Could you check a few things on this model? Use its own coordinates, in mm. Face numbers are marked on the shaded views. Round coordinates to 2 decimals unless told otherwise and drop trailing zeros. Write each loop counter-clockwise with the first axis right and the second up, starting at its lowest first coordinate (ties: lowest second). Pieces come first, ordered by that corner, then holes. Notation, with made-up numbers: (8, -19) -> (45, -19) arc R26 cw to (45, 15) -> close; hole circle Ø8 at (66, -34.75). An arc over 180 degrees is marked (long way). One line per question, with ' | ' between items. Start each with the question number.
1. Imagine slicing it at C-C, the plane x = 0. State how many separate pieces and enclosed holes the cut face has, and give its area (3 significant figures).
2. Imagine slicing it at D-D, the plane x = -7.75. List the corners of the cut face in (y, z) for me.
3. For pin 1 Ø4 at (x, y) = (-5, 25) entering from -Z; pin 2 Ø4 at (x, z) = (1.5, 22.5) entering from +Y; pin 3 Ø10 at (y, z) = (3.5, -17) entering from +X; pin 4 Ø2.5 at (x, z) = (0, 20) entering from +Y, each with a flat end and sliding along its axis, tell me the tip position at first contact or that it passes through.
4. Imagine slicing it at A-A, the plane z = 0. List the corners of the cut face in (x, y) for me (3 decimals), and give its area (4 significant figures).
5. Imagine slicing it at B-B, the plane y = 15.5. List the corners of the cut face in (x, z) for me.
6. If I drill on line 1 along Z through (x, y) = (0, 28.95) (3 decimals); line 2 along Z through (x, y) = (0, 2.2); line 3 along X through (y, z) = (4.5, -19), over which ranges is the centre line in solid material (lowest first)? Write a range as [from, to].
7. Thinking about a two-plate mould opening in Z: for the marked faces 1, 2, 3 and 4, which applies, released by +Z, released by -Z, zero draft, split by the parting line, or undercut?
Autodesk Inventor part; units mm, degrees
ref_plane "YZ Plane" through (0, 0, 0) normal (1, 0, 0) x (0, 1, 0)
ref_plane "XZ Plane" through (0, 0, 0) normal (0, 1, 0) x (-1, 0, 0)
ref_plane "XY Plane" through (0, 0, 0) normal (0, 0, 1) x (1, 0, 0)
sketch "スケッチ1" plane through (0, 0, 0) normal (0, 1, 0) x (-1, 0, 0)
  line L0 (0, 0) -> (0, -20) construction
  line L1 (0, 0) -> (0, 20) construction
  circle A0 centre (0, 20) radius 1.7
  circle A1 centre (0, -20) radius 1.7
  circle A2 centre (0, 20) radius 4.7
  circle A3 centre (0, -20) radius 4.7
  line L2 (4.698231, 19.871077) -> (4.7, -19.999792)
  line L3 (-4.697377, 19.843003) -> (-4.697377, -20.156997)
  circle A4 centre (0, 0) radius 12.5
  point P0 (-4.697377, 11.58381)
  point P1 (4.698599, 11.583314)
  point P2 (4.699627, -11.582897)
  point P3 (-4.697377, -11.58381)
  dimension "d0" = 20
  dimension "d1" = 20
  dimension "d2" = 3.4
  dimension "d3" = 3.4
  dimension "d5" = 3
  dimension "d6" = 3
  dimension "d7" = 25
sketch "スケッチ1 outline for 押し出し1" plane through (0, 0, 0) normal (0, 1, 0) x (-1, 0, 0)
  arc A0 (-4.697377, 11.58381) -> (4.698599, 11.583314) centre (0, 0) cw
  line L0 (-4.697377, 19.843003) -> (-4.697377, 11.58381)
  line L1 (4.698599, 11.583314) -> (4.698231, 19.871077)
  arc A1 (4.698231, 19.871077) -> (-4.697377, 19.843003) centre (0, 20) ccw
  circle A2 centre (0, 20) radius 1.7
  arc A3 (-4.697377, -20.156997) -> (4.7, -19.999792) centre (0, -20) ccw
  line L2 (-4.697377, -11.58381) -> (-4.697377, -20.156997)
  line L3 (4.7, -19.999792) -> (4.699627, -11.582897)
  arc A4 (4.699627, -11.582897) -> (-4.697377, -11.58381) centre (0, 0) cw
  circle A5 centre (0, -20) radius 1.7
extrude "押し出し1" add sketch "スケッチ1 outline for 押し出し1" along normal blind 5
sketch "スケッチ2" plane through (0, 5, 0) normal (0, 1, 0) x (1, 0, 0)
  line L0 (-4.698599, -11.583314) -> (-4.698231, -19.871077)
  arc A0 (-4.698231, -19.871077) -> (4.697377, -19.843003) centre (0, -20) ccw
  line L1 (4.697377, -19.843003) -> (4.697377, -11.58381)
  arc A1 (-4.698599, -11.583314) -> (4.697377, -11.58381) centre (0, 0) ccw
  circle A2 centre (0, -20) radius 1.7
  arc A3 (4.697377, 20.156997) -> (-4.7, 19.999792) centre (0, 20) ccw
  line L2 (-4.7, 19.999792) -> (-4.699627, 11.582897)
  arc A4 (4.697377, 11.58381) -> (-4.699627, 11.582897) centre (0, 0) ccw
  line L3 (4.697377, 11.58381) -> (4.697377, 20.156997)
  circle A5 centre (0, 20) radius 1.7
  circle A6 centre (0, 0) radius 16
  point P0 (4.697377, 15.294922)
  point P1 (-4.699791, 15.294181)
  point P2 (-4.698434, -15.294598)
  point P3 (4.697377, -15.294922)
  dimension "d10" = 32
extrude "押し出し2" add sketch "スケッチ2" along normal blind 20 contours A1 L1 A6 L0 | A6 L3 A4 L2
sketch "スケッチ3" plane through (0, 25, 0) normal (0, 1, 0) x (1, 0, 0)
  line L0 (-4.698599, -11.583314) -> (-4.698434, -15.294598)
  arc A0 (-4.698434, -15.294598) -> (4.697377, -15.294922) centre (0, 0) ccw
  line L1 (4.697377, -15.294922) -> (4.697377, -11.58381)
  arc A1 (-4.698599, -11.583314) -> (4.697377, -11.58381) centre (0, 0) ccw
  line L2 (-4.699791, 15.294181) -> (-4.699627, 11.582897)
  arc A2 (4.697377, 11.58381) -> (-4.699627, 11.582897) centre (0, 0) ccw
  line L3 (4.697377, 11.58381) -> (4.697377, 15.294922)
  arc A3 (4.697377, 15.294922) -> (-4.699791, 15.294181) centre (0, 0) ccw
  line L4 (-4.6, -11.583314) -> (-4.6, 11.582897)
  line L5 (4.697377, -11.58381) -> (4.697377, 11.58381)
  circle A4 centre (0, 0) radius 10
  point P0 (-4.699504, 8.826928)
  point P1 (-4.698721, -8.827345)
  point P2 (4.697377, -8.82806)
  point P3 (4.697377, 8.82806)
  dimension "d16" = 20
sketch "スケッチ3 outline for 押し出し3" plane through (0, 25, 0) normal (0, 1, 0) x (1, 0, 0)
  arc A0 (4.697377, 15.294922) -> (-4.699791, 15.294181) centre (0, 0) ccw
  line L0 (-4.699791, 15.294181) -> (-4.699504, 8.826928)
  arc A1 (-4.699504, 8.826928) -> (-4.698721, -8.827345) centre (0, 0) ccw
  line L1 (-4.698721, -8.827345) -> (-4.698434, -15.294598)
  arc A2 (-4.698434, -15.294598) -> (4.697377, -15.294922) centre (0, 0) ccw
  line L2 (4.697377, -15.294922) -> (4.697377, -8.82806)
  arc A3 (4.697377, -8.82806) -> (4.697377, 8.82806) centre (0, 0) ccw
  line L3 (4.697377, 8.82806) -> (4.697377, 15.294922)
extrude "押し出し3" add sketch "スケッチ3 outline for 押し出し3" along normal blind 5
sketch "スケッチ5" plane through (0, 30, 0) normal (0, 1, 0) x (1, 0, 0)
  circle A0 centre (0, 0) radius 6
  line L0 (0, 0) -> (0, 9)
  line L1 (0, 9) -> (0, -9)
  dimension "d18" = 12
  dimension "d19" = 9
  dimension "d20" = 18
hole "穴1" at (0, 30, -9) at (0, 30, 9) direction (0, -1, 0) diameter 3.4 end through all
sketch "スケッチ6" plane through (0, 30, 0) normal (0, 1, 0) x (1, 0, 0)
  point P0 (0, 0)
  point P1 (0, 0)
hole "穴2" at (0, 30, 0) direction (0, -1, 0) diameter 12.35 end through all
fillet "フィレット3" radius 2 4 edges at (-4.6987, 27.5, 8.8273) (-4.6995, 27.5, -8.8269) (4.6974, 27.5, 8.8281) (4.6974, 27.5, -8.8281)
fillet "フィレット4" radius 1 6 edges at (-0.0006, 30, 16) (-0.0013, 30, -16) (-0.0007, 0, 12.5) (-0.0012, 0, -12.5) (-0.0006, 5, 16) (-0.0013, 5, -16)
properties part number "Th_3D_hn_1" material "ABS プラスチック"
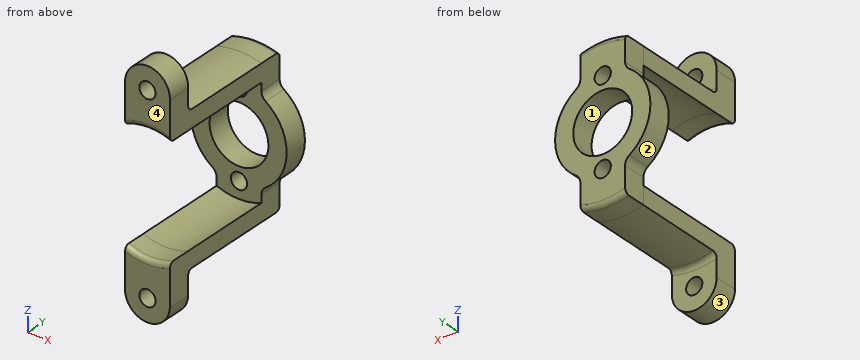
Geometry results:
1) separate pieces: 6 | enclosed holes: 0 | area: 292 mm2
2) outline: (25, -6.32) -> (30, -6.32) -> (30, 6.32) -> (25, 6.32) -> close
3) pin 1: stops at z = -15.72 | pin 2: stops at y = 5 | pin 3: stops at x = 4.7 | pin 4: passes through
4) outline: (-10, 25) -> (-6.175, 25) -> (-6.175, 30) -> (-10, 30) -> close; (6.175, 25) -> (10, 25) -> (10, 30) -> (6.175, 30) -> close | area: 38.25 mm2
5) outline: (-4.7, -15.29) arc R16 ccw to (4.7, -15.29) -> (4.7, -11.58) arc R12.5 cw to (-4.7, -11.58) -> close; (-4.7, 11.58) arc R12.5 cw to (4.7, 11.58) -> (4.7, 15.29) arc R16 ccw to (-4.7, 15.29) -> close
6) line 1: z = [-16, -10.7], [-7.3, -6.175], [6.175, 7.3], [10.7, 16] | line 2: z = [-24.7, -21.7], [-18.3, -12.5], [12.5, 18.3], [21.7, 24.7] | line 3: x = [-4.7, -1.37], [1.37, 4.7]
7) face 1: undercut | face 2: split by the parting line | face 3: released by -Z | face 4: zero draft
